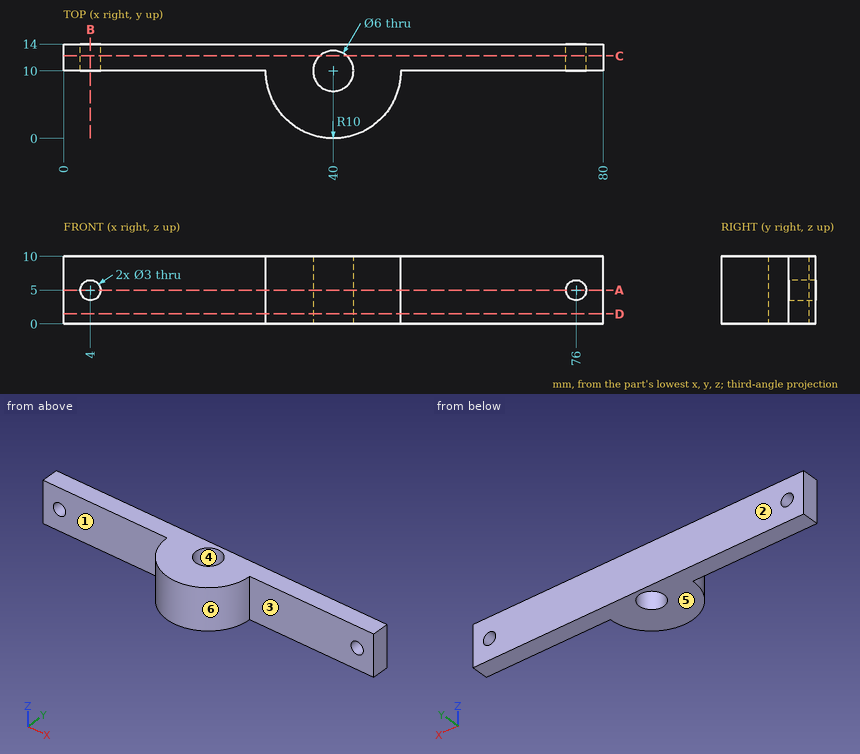
The figure shows three views and two pictorial views of one solid part (mm, origin at its lowest corner). Answer the questions. A direction names the side the tool comes from. Round coordinates to 2 decimals unless told otherwise and drop trailing zeros. Order: outer loops, then holes, each group sorted by start corner. A loop starts at its lowest first (then second) coordinate and runs counter-clockwise, first axis right, second up. Notation, with made-up numbers: M 86,77 L 137,77 A28 cw 137,102 Z; hole C 29,14 d7. An arc over 180 degrees is marked long. Answer in a Markdown table with one row per item. Add a question column.
1) The part is cut by section A-A on z = 5. Determine the outline of the cut face in (x, y), plus the area to 3 significant figures.
2) Flat-ended cylindrical pins translate along their axes: pin 1 Ø6 at (y, z) = (3, 7) entering from -X; pin 2 Ø5 at (x, y) = (40, 10) entering from +Z; pin 3 Ø1 at (y, z) = (9, 7.5) entering from +X; pin 4 Ø3 at (x, z) = (22, 3.5) entering from -Y. Find the tip coordinate at first contact, or state that the pin passes through.
3) Determine the mould class of the marked faces 4, 5 and 6 for opening direction X: pulls with the +X half, pulls with the -X half, needs draft (parallel to the pull), parting line crosses it, or undercut.
4) The part is cut by section B-B on x = 4. Determine the outline of the cut face in (y, z).
5) The part is cut by section D-D on z = 1.5. Determine the outline of the cut face in (x, y).
6) Consider line 1 along X through (y, z) = (13.15, 5); line 2 along Y through (x, z) = (40, 3.25); line 3 along X through (y, z) = (12.65, 5). Determine where each line is inside the solid, lowest interval first. Write a range as from..to.
7) The part is cut by section C-C on y = 12.25. Determine the outline of the cut face in (x, z).
8) Which of the six approach directions +Z, -Z, +X, -X, +Y, -Y give full straight-line access (tool end or side, diameter ignored) to the marked faces 1, 2 and 3?
Findings below:
| question | item | result |
|---|---|---|
| 1 | outline | M 0,10 L 2.5,10 L 2.5,14 L 0,14 Z; M 5.5,10 L 30,10 A10 ccw 50,10 L 74.5,10 L 74.5,14 L 5.5,14 Z; M 77.5,10 L 80,10 L 80,14 L 77.5,14 Z; hole C 40,10 d6 |
| 1 | area | 425 mm² |
| 2 | pin 1 | stops at x = 30.83 |
| 2 | pin 2 | passes through |
| 2 | pin 3 | stops at x = 49.99 |
| 2 | pin 4 | stops at y = 10 |
| 3 | face 4 | undercut |
| 3 | face 5 | needs draft |
| 3 | face 6 | parting line crosses it |
| 4 | outline | M 10,0 L 14,0 L 14,3.5 L 10,3.5 Z; M 10,6.5 L 14,6.5 L 14,10 L 10,10 Z |
| 5 | outline | M 0,10 L 30,10 A10 ccw 50,10 L 80,10 L 80,14 L 0,14 Z; hole C 40,10 d6 |
| 6 | line 1 | x = 0..2.5, 5.5..74.5, 77.5..80 |
| 6 | line 2 | y = 0..7, 13..14 |
| 6 | line 3 | x = 0..2.5, 5.5..38.59, 41.41..74.5, 77.5..80 |
| 7 | outline | M 0,0 L 38.02,0 L 38.02,10 L 0,10 Z; M 41.98,0 L 80,0 L 80,10 L 41.98,10 Z; hole C 4,5 d3; hole C 76,5 d3 |
| 8 | face 1 | +Z, -Z, -X, -Y |
| 8 | face 2 | +Z, -Z, +X, -X, +Y |
| 8 | face 3 | +Z, -Z, +X, -Y |
